Here's how the part is built. I have some questions about the finished solid (model axes, mm). A direction names the side the tool comes from. Round coordinates to 2 decimals unless told otherwise and drop trailing zeros. Write each loop counter-clockwise with the first axis right and the second up, starting at its lowest first coordinate (ties: lowest second). Pieces come first, ordered by that corner, then holes. Notation, with made-up numbers: (51, 63.5) -> (81, 63.5) arc R26 cw to (81, 98.5) -> close; hole circle Ø6 at (-4.75, 71). An arc over 180 degrees is marked (long way). Put each result on its own line as item: value. Start each with the question number.
1) I want a section at A-A, the plane y = -36. List the corners of the cut face in (x, z) for me.
2) Which directions (+Z, -Z, +X, -X, +Y, -Y) give clear straight access to the entire face, cutting with the end or side of a thin tool? Please do faces 1 (the cylindrical face through (-2.38, -50.03, -10.74)), 2 (the flat face through (-7.89, 7.16, 13.92)), 3 (the flat face through (0, 0.5, -17)), 4 (the flat face through (-14.4, 0.5, -8.4)).
3) If I drill on line 1 along X through (y, z) = (-15, 0); line 2 along Y through (x, z) = (-11, 10.5); line 3 along X through (y, z) = (-1.5, 6), over which ranges is the centre line in solid material (lowest first)? Write a range as [from, to].
4) Will these pins go through, and if not, where does the flat tip stop? P1, Ø10, axis at y = -34, z = 13.5, coming from the -X side; P2, Ø8, axis at y = -65.5, z = -4.5, coming from the +X side; P3, Ø5, axis at x = -12, y = -39, coming from the -Z side; P4, Ø1, axis at y = -69, z = -13, coming from the +X side.
Autodesk Inventor part; units mm, degrees
ref_plane "YZ Plane" through (0, 0, 0) normal (1, 0, 0) x (0, 1, 0)
ref_plane "XZ Plane" through (0, 0, 0) normal (0, 1, 0) x (-1, 0, 0)
ref_plane "XY Plane" through (0, 0, 0) normal (0, 0, 1) x (1, 0, 0)
sketch "Sketch1" plane through (0, 0, 0) normal (0, 1, 0) x (-1, 0, 0)
  line L0 (127.8939, 73.8396) -> (127.8939, -73.8396)
  line L1 (127.8939, -73.8396) -> (0, -147.6791)
  line L2 (0, -147.6791) -> (-127.8939, -73.8396)
  line L3 (-127.8939, -73.8396) -> (-127.8939, 73.8396)
  line L4 (-127.8939, 73.8396) -> (0, 147.6791)
  line L5 (0, 147.6791) -> (127.8939, 73.8396)
  line L6 (-16, 9.2376) -> (0, 18.4752)
  line L7 (0, 18.4752) -> (16, 9.2376)
  line L8 (16, 9.2376) -> (16, -9.2376)
  line L9 (16, -9.2376) -> (0, -18.4752)
  line L10 (0, -18.4752) -> (-16, -9.2376)
  line L11 (-16, -9.2376) -> (-16, 9.2376)
  point P0 (0, 0)
  point P1 (0, 0)
  point P2 (0, 0)
  dimension "Shex" = 32
extrude "Extrusion1" add sketch "Sketch1" along normal blind 14 contours L6 L7 L8 L9 L10 L11
sketch "Sketch2" plane through (0, 0, 0) normal (1, 0, 0) x (0, 1, 0)
  line L0 (0, -18.4752) -> (14, -18.4752) construction
  line L1 (14, -18.4752) -> (12.5709, -18.4752)
  line L2 (12.5709, -18.4752) -> (14, -16)
  line L3 (14, -16) -> (14, -18.4752)
  line L4 (-3, 0) -> (18, 0)
  point P0 (0, 0)
  dimension "d4" = 60
  dimension "d5" = 32
revolve "Revolution1" cut sketch "Sketch2" angle 360 about axis through (0, -10, 0) along (0, 1, 0)
sketch "Sketch3" plane through (0, 0, 0) normal (0, 0, 1) x (1, 0, 0)
  line L0 (0, 0) -> (11, 0)
  line L1 (11, 0) -> (11, -100)
  line L2 (11, -100) -> (0, -100)
  line L3 (0, -100) -> (0, 0)
  dimension "L" = 100
  dimension "Dia" = 22
revolve "Revolution2" add sketch "Sketch3" angle 360 about axis through (0, -100, 0) along (0, 1, 0)
fillet "Fillet1" radius 0.7 1 edges at (-11, 0, 0)
chamfer "Chamfer1" distance 2 angle 45 1 edges at (-11, -100, 0)
thread "Thread2"
sketch "Sketch6" plane through (0, 0, 0) normal (1, 0, 0) x (0, 1, 0)
  line L0 (-3.0757, 0) -> (18.4544, 0)
  line L1 (0, -18.4752) -> (12.5709, -18.4752)
  line L2 (0, -18.4752) -> (0, -9.2376)
  line L3 (0, -9.2376) -> (12.5709, -9.2376)
  line L4 (0, -18.4752) -> (0.5, -18.4752)
  line L5 (0.5, -18.4752) -> (0.5, -16)
  line L6 (0.5, -16) -> (0, -16)
  line L7 (0, -16) -> (0, -18.4752)
  point P0 (0, 0)
  point P1 (14, -13.8564)
  point P2 (0, -16)
  dimension "a" = 0.5
  dimension "d34" = 32
revolve "Revolution3" cut sketch "Sketch6" angle 360 about axis through (0, -10, 0) along (0, 1, 0)
equation "\"d5\" = Shex"
equation "\"d31\" = b - cham"
equation "\"d34\" = Shex"
equation "\"b\" = 54"
properties part number "SCREW M24x120-01-02" material "Steel"
Findings:
1. outline: circle Ø22 at (0, 0)
2. face 1: -Y
2. face 2: +Z, -X, +Y, -Y
2. face 3: -Z, -Y
2. face 4: -Z, -X, -Y
3. line 1: x = [-11, 11]
3. line 2: y = [0, 14]
3. line 3: x = [-9.22, 9.22]
4. P1: stops at x = -6.98
4. P2: stops at x = 10.99
4. P3: stops at z = -5.55
4. P4: passes through
